```python
from build123d import *

# Parameters (mm, degrees)
MODEL_R                 = 1.5
MODEL_R_2               = 2.2
P_IDAT_VYSUNUT_M1_DEPTH = 2.8


with BuildPart() as part:
    # Model → Přidat vysunutím1 (new body)
    with BuildSketch(Plane.XY):
        with BuildLine():
            Line((-14.2, 18.25), (14.2, 18.25))
            Line((14.2, 18.25), (15.610615846, 10.25))
            Line((15.610615846, 10.25), (16.010615846, 10.25))
            Line((16.010615846, 10.25), (14.071019058, 21.25))
            Line((14.071019058, 21.25), (12.101403552, 20.902703645))
            Line((12.101403552, 20.902703645), (11.893025739, 22.084472948))
            Line((11.893025739, 22.084472948), (14.706771698, 23.907401431))
            Line((14.706771698, 23.907401431), (15.892964362, 24.088914415))
            Line((15.892964362, 24.088914415), (18.010615846, 10.25))
            Line((18.010615846, 10.25), (18.9, 10.25))
            Line((18.9, 10.25), (18.9, 21.596640106))
            ThreePointArc((18.9, 21.596640106), (20.7, 22.05), (22.5, 21.596640106))
            Line((22.5, 21.596640106), (22.5, 10.25))
            Line((22.5, 10.25), (23.389384154, 10.25))
            Line((23.389384154, 10.25), (25.507035638, 24.088914415))
            Line((25.507035638, 24.088914415), (26.693228302, 23.907401431))
            Line((26.693228302, 23.907401431), (29.506974261, 22.084472948))
            Line((29.506974261, 22.084472948), (29.298596448, 20.902703645))
            Line((29.298596448, 20.902703645), (27.328980942, 21.25))
            Line((27.328980942, 21.25), (25.389384154, 10.25))
            Line((25.389384154, 10.25), (25.789384154, 10.25))
            Line((25.789384154, 10.25), (27.2, 18.25))
            Line((27.2, 18.25), (32.5, 18.25))
            Line((32.5, 18.25), (32.5, -18.25))
            Line((32.5, -18.25), (27.2, -18.25))
            Line((27.2, -18.25), (25.789384154, -10.25))
            Line((25.789384154, -10.25), (25.389384154, -10.25))
            Line((25.389384154, -10.25), (27.328980942, -21.25))
            Line((27.328980942, -21.25), (29.298596448, -20.902703645))
            Line((29.298596448, -20.902703645), (29.506974261, -22.084472948))
            Line((29.506974261, -22.084472948), (26.693228302, -23.907401431))
            Line((26.693228302, -23.907401431), (25.507035638, -24.088914415))
            Line((25.507035638, -24.088914415), (23.389384154, -10.25))
            Line((23.389384154, -10.25), (22.5, -10.25))
            Line((22.5, -10.25), (22.5, -21.596640106))
            ThreePointArc((22.5, -21.596640106), (20.7, -22.05), (18.9, -21.596640106))
            Line((18.9, -21.596640106), (18.9, -10.25))
            Line((18.9, -10.25), (18.010615846, -10.25))
            Line((18.010615846, -10.25), (15.892964362, -24.088914415))
            Line((15.892964362, -24.088914415), (14.706771698, -23.907401431))
            Line((14.706771698, -23.907401431), (11.893025739, -22.084472948))
            Line((11.893025739, -22.084472948), (12.101403552, -20.902703645))
            Line((12.101403552, -20.902703645), (14.071019058, -21.25))
            Line((14.071019058, -21.25), (16.010615846, -10.25))
            Line((16.010615846, -10.25), (15.610615846, -10.25))
            Line((15.610615846, -10.25), (14.2, -18.25))
            Line((14.2, -18.25), (3.5, -18.25))
            Line((3.5, -18.25), (3.5, -12.45))
            Line((3.5, -12.45), (-3.5, -12.45))
            Line((-3.5, -12.45), (-3.5, -18.25))
            Line((-3.5, -18.25), (-14.2, -18.25))
            Line((-14.2, -18.25), (-15.610615846, -10.25))
            Line((-15.610615846, -10.25), (-16.010615846, -10.25))
            Line((-16.010615846, -10.25), (-14.071019058, -21.25))
            Line((-14.071019058, -21.25), (-12.101403552, -20.902703645))
            Line((-12.101403552, -20.902703645), (-11.893025739, -22.084472948))
            Line((-11.893025739, -22.084472948), (-14.706771698, -23.907401431))
            Line((-14.706771698, -23.907401431), (-15.892964362, -24.088914415))
            Line((-15.892964362, -24.088914415), (-18.010615846, -10.25))
            Line((-18.010615846, -10.25), (-18.9, -10.25))
            Line((-18.9, -10.25), (-18.9, -21.596640106))
            ThreePointArc((-18.9, -21.596640106), (-20.7, -22.05), (-22.5, -21.596640106))
            Line((-22.5, -21.596640106), (-22.5, -10.25))
            Line((-22.5, -10.25), (-23.389384154, -10.25))
            Line((-23.389384154, -10.25), (-25.507035638, -24.088914415))
            Line((-25.507035638, -24.088914415), (-26.693228302, -23.907401431))
            Line((-26.693228302, -23.907401431), (-29.506974261, -22.084472948))
            Line((-29.506974261, -22.084472948), (-29.298596448, -20.902703645))
            Line((-29.298596448, -20.902703645), (-27.328980942, -21.25))
            Line((-27.328980942, -21.25), (-25.389384154, -10.25))
            Line((-25.389384154, -10.25), (-25.789384154, -10.25))
            Line((-25.789384154, -10.25), (-27.2, -18.25))
            Line((-27.2, -18.25), (-32.5, -18.25))
            Line((-32.5, -18.25), (-32.5, 18.25))
            Line((-32.5, 18.25), (-27.2, 18.25))
            Line((-27.2, 18.25), (-25.789384154, 10.25))
            Line((-25.789384154, 10.25), (-25.389384154, 10.25))
            Line((-25.389384154, 10.25), (-27.328980942, 21.25))
            Line((-27.328980942, 21.25), (-29.298596448, 20.902703645))
            Line((-29.298596448, 20.902703645), (-29.506974261, 22.084472948))
            Line((-29.506974261, 22.084472948), (-26.693228302, 23.907401431))
            Line((-26.693228302, 23.907401431), (-25.507035638, 24.088914415))
            Line((-25.507035638, 24.088914415), (-23.389384154, 10.25))
            Line((-23.389384154, 10.25), (-22.5, 10.25))
            Line((-22.5, 10.25), (-22.5, 21.596640106))
            ThreePointArc((-22.5, 21.596640106), (-20.7, 22.05), (-18.9, 21.596640106))
            Line((-18.9, 21.596640106), (-18.9, 10.25))
            Line((-18.9, 10.25), (-18.010615846, 10.25))
            Line((-18.010615846, 10.25), (-15.892964362, 24.088914415))
            Line((-15.892964362, 24.088914415), (-14.706771698, 23.907401431))
            Line((-14.706771698, 23.907401431), (-11.893025739, 22.084472948))
            Line((-11.893025739, 22.084472948), (-12.101403552, 20.902703645))
            Line((-12.101403552, 20.902703645), (-14.071019058, 21.25))
            Line((-14.071019058, 21.25), (-16.010615846, 10.25))
            Line((-16.010615846, 10.25), (-15.610615846, 10.25))
            Line((-15.610615846, 10.25), (-14.2, 18.25))
        make_face()
        with Locations((-8.75, 13.25)):
            Circle(MODEL_R, mode=Mode.SUBTRACT)
        with Locations(Location((8.75, 13.25, 0), (0, 0, 180))):
            Circle(MODEL_R_2, mode=Mode.SUBTRACT)
        with BuildLine():
            Line((2.875009535, -8.806924836), (5.5, 0))
            Line((5.5, 0), (3, 0))
            ThreePointArc((3, 0), (0, 3), (-3, 0))
            Line((-3, 0), (-5.5, 0))
            Line((-5.5, 0), (-2.875009535, -8.806924836))
            ThreePointArc((-2.875009535, -8.806924836), (0, -10.95), (2.875009535, -8.806924836))
        make_face(mode=Mode.SUBTRACT)
    extrude(amount=P_IDAT_VYSUNUT_M1_DEPTH)


solid = part.part
```
For this review, take the finished solid that the model builds, in its own axes (mm). A direction names the side the tool comes from. Round coordinates to 2 decimals unless told otherwise and drop trailing zeros. Write each loop counter-clockwise with the first axis right and the second up, starting at its lowest first coordinate (ties: lowest second). Pieces come first, ordered by that corner, then holes. Notation, with made-up numbers: M -26.5,46.5 L 7.5,46.5 A14 cw 7.5,61.5 Z; hole C -32.5,21 d1. An arc over 180 degrees is marked long. One line per item, written item: value. Start each with the question number.
(1) Wall thickness on line 1 (Y direction, x = -8.75, z = 0.9); line 2 (X direction, y = -3, z = 0.65); line 3 (Y direction, x = -6, z = 0.95): over which ranges is each line inside the solid? List them lowest first.
(2) The part is to be moulded in two halves that separate along X. For faces 1 (the flat face through (-30, -18.25, 1)), 2 (the flat face through (-28.12, 22.983, 1.38)), 3 (the flat face through (0, -12.45, 1)), say which applies: released by +X, released by -X, zero draft, split by the parting line, or undercut.
(3) Insertion check: pin 1 (1.4 mm diameter, centred on x = -29.5, z = 1, fed in from -Y); pin 2 (1.5 mm diameter, centred on x = -9, z = 1.5, fed in from -Y); pin 3 (1.4 mm diameter, centred on x = 30, z = 1, fed in from +Y). Each pin has a flat end and moves straight along its axis. Give the tip position at first contact, or say it passes through.
(4) Machinability: for faces 4 (the flat face through (-18.9, 16, 1)), 5 (the flat face through (15.054, 15.673, 1.38)), 6 (the flat face through (-22.5, -16, 1)), which of the approach directions +Z, -Z, +X, -X, +Y, -Y give a long, thin tool a straight path to every point of the face, cutting with its end or side? Answer none if there is none.
(5) We need section B-B (x = 0). Give the boundary of the cut face in (y, z), and give its area (3 significant figures).
(6) We need section C-C (y = 13.25). Count the separate pieces of the cut face and the enclosed holes in it, and give its area (3 significant figures).
(7) We need section A-A (x = -8.75). Give the boundary of the cut face in (y, z), and give its area (3 significant figures).
Result:
1. line 1: -18.25 to 11.75, 14.75 to 18.25
1. line 2: -32.5 to -4.61, 4.61 to 32.5
1. line 3: -18.25 to 18.25
2. face 1: zero draft
2. face 2: released by -X
2. face 3: undercut
3. pin 1: y = -22.54
3. pin 2: y = -18.25
3. pin 3: y = 22.22
4. face 4: +Z, -Z, +Y
4. face 5: +Z, -Z
4. face 6: +Z, -Z, -Y
5. outline: M -12.45,0 L -10.95,0 L -10.95,2.8 L -12.45,2.8 Z; M 3,0 L 18.25,0 L 18.25,2.8 L 3,2.8 Z
5. area: 46.9 mm²
6. separate pieces: 11
6. enclosed holes: 0
6. area: 142 mm²
7. outline: M -18.25,0 L 11.75,0 L 11.75,2.8 L -18.25,2.8 Z; M 14.75,0 L 18.25,0 L 18.25,2.8 L 14.75,2.8 Z
7. area: 93.8 mm²
